Autodesk Inventor part; units mm, degrees
ref_plane "YZ Plane" through (0, 0, 0) normal (1, 0, 0) x (0, 1, 0)
ref_plane "XZ Plane" through (0, 0, 0) normal (0, 1, 0) x (-1, 0, 0)
ref_plane "XY Plane" through (0, 0, 0) normal (0, 0, 1) x (1, 0, 0)
sketch "Sketch1" plane through (0, 0, 0) normal (0, 0, 1) x (1, 0, 0)
  line L0 (-12.7, -25.4) -> (12.7, -25.4)
  line L1 (12.7, -25.4) -> (12.7, 25.4)
  line L2 (12.7, 25.4) -> (-12.7, 25.4)
  line L3 (-12.7, 25.4) -> (-12.7, -25.4)
  line L4 (-12.7, -25.4) -> (12.7, 25.4) construction
  line L5 (12.7, -25.4) -> (-12.7, 25.4) construction
  line L6 (-11.1125, 23.8125) -> (11.1125, 23.8125)
  line L7 (11.1125, 23.8125) -> (11.1125, -23.8125)
  line L8 (11.1125, -23.8125) -> (-11.1125, -23.8125)
  line L9 (-11.1125, -23.8125) -> (-11.1125, 23.8125)
  point P0 (0, 0)
  dimension "width" = 25.4
  dimension "height" = 50.8
  dimension "thickness" = 1.5875
extrude "Extrusion1" add sketch "Sketch1" along normal mid plane 914.4
sketch "Sketch2" plane through (-12.7, 25.4, 457.2) normal (0, 1, 0) x (1, 0, 0)
  line L0 (25.4, 0) -> (0, 0)
  line L1 (0, 914.4) -> (0, 0)
  point P0 (12.7, 457.2)
  point P1 (12.7, 6.35)
  point P2 (12.7, 12.7)
  point P3 (12.7, 19.05)
  point P4 (12.7, 0)
  point P5 (12.7, 0)
  dimension "d5" = 6.35
  dimension "d6" = 6.35
  dimension "d7" = 6.35
hole "Hole1" at (0, 25.4, 450.85) at (0, 25.4, 444.5) at (0, 25.4, 438.15) direction (0, -1, 0) diameter 5.1054 end through all
sketch "Sketch3" plane through (-12.7, -25.4, 457.2) normal (-1, 0, 0) x (0, 0, 1)
  line L0 (-914.4, 0) -> (-914.4, 50.8)
  point P0 (-457.2, 25.4)
  point P1 (-901.7, 38.1)
  point P2 (-901.7, 25.4)
  point P3 (-901.7, 12.7)
  point P4 (-914.4, 25.4)
  dimension "d15" = 12.7
  dimension "d16" = 12.7
  dimension "d17" = 12.7
hole "Hole2" at (-12.7, 12.7, -444.5) at (-12.7, 0, -444.5) at (-12.7, -12.7, -444.5) direction (1, 0, 0) diameter 5.1054 end through all
sketch "Sketch4" plane through (-12.7, 25.4, 457.2) normal (0, 1, 0) x (1, 0, 0)
  circle A0 centre (12.7, 19.05) radius 2.5527
  line L0 (25.4, 914.4) -> (25.4, 0)
  point P0 (12.7, 457.2)
  point P1 (15.4686, 44.45)
  dimension "d34" = 9.9314
  dimension "d55" = 25.4
hole "Hole3" at (2.7686, 25.4, 412.75) direction (0, -1, 0) diameter 9.525 end through all
sketch "Sketch5" plane through (-12.7, 25.4, 457.2) normal (0, 1, 0) x (1, 0, 0)
  line L0 (0, 914.4) -> (25.4, 914.4)
  line L1 (0, 914.4) -> (0, 0)
  point P0 (12.7, 457.2)
  point P1 (9.9314, 869.95)
  point P2 (12.7, 914.4)
  dimension "d35" = 44.45
  dimension "d36" = 9.9314
hole "Hole4" at (-2.7686, 25.4, -412.75) direction (0, -1, 0) diameter 9.525 end through all
sketch "Sketch6" plane through (12.7, -25.4, 457.2) normal (1, 0, 0) x (0, 0, -1)
  line L0 (58.42, 41.275) -> (30.48, 41.275)
  line L1 (30.48, 41.275) -> (30.48, 9.525)
  line L2 (30.48, 9.525) -> (58.42, 9.525)
  line L3 (58.42, 9.525) -> (58.42, 41.275)
  line L4 (58.42, 41.275) -> (30.48, 9.525) construction
  line L5 (30.48, 41.275) -> (58.42, 9.525) construction
  line L6 (0, 0) -> (0, 50.8)
  line L7 (914.4, 50.8) -> (0, 50.8)
  point P0 (457.2, 25.4)
  point P1 (44.45, 25.4)
  point P2 (0, 25.4)
  dimension "d44" = 30.48
  dimension "d45" = 27.94
  dimension "d47" = 31.75
extrude "Extrusion2" cut sketch "Sketch6" against normal blind 1.5875
sketch "Sketch7" plane through (-12.7, -25.4, 457.2) normal (-1, 0, 0) x (0, 0, 1)
  line L0 (-883.92, 9.525) -> (-855.98, 9.525)
  line L1 (-855.98, 9.525) -> (-855.98, 41.275)
  line L2 (-855.98, 41.275) -> (-883.92, 41.275)
  line L3 (-883.92, 41.275) -> (-883.92, 9.525)
  line L4 (-883.92, 9.525) -> (-855.98, 41.275) construction
  line L5 (-855.98, 9.525) -> (-883.92, 41.275) construction
  line L6 (-914.4, 0) -> (-914.4, 50.8)
  point P0 (-457.2, 25.4)
  point P1 (-869.95, 25.4)
  point P2 (-914.4, 25.4)
  dimension "d50" = 30.48
  dimension "d51" = 31.75
  dimension "d52" = 27.94
extrude "Extrusion3" cut sketch "Sketch7" against normal blind 1.5875
properties part number "EL2-004" material "Aluminum 6061"
Work out the finished part from the listing and answer in its coordinate system (mm). A direction names the side the tool comes from. Give positions to 0.01 mm unless a question says otherwise; leave off trailing zeros. Write each loop counter-clockwise with the first axis right and the second up, starting at its lowest first coordinate (ties: lowest second). Pieces come first, ordered by that corner, then holes.
Q1. For a pull along Y with two mould halves and no side action, classify faces 1 (the face through (0, 25.4, -6)), 2 (the face through (-11.3, 2, -457.2)), 3 (the face through (-11.112, 0, -6)) as released by +Y, released by -Y, zero draft, split by the parting line, or undercut.
Answer:
face 1: released by +Y
face 2: zero draft
face 3: undercut
Q2. A tool of negligible diameter and unlimited length cuts with its end or side. For faces 4 (the face through (-11.3, 2, 457.2)), 5 (the face through (11.112, 0, -6)), from which of +Z, -Z, +X, -X, +Y, -Y can it reach the whole face along a straight path? Write none if from no direction.
Answer:
face 4: +Z, +X, -X, +Y, -Y
face 5: +Z, -Z
Q3. Straight lines are drawn through the part: L1, parallel to Z at x = -12.1, y = 0; L2, parallel to Z at x = 11.5, y = -12.7; L3, parallel to Y at x = -11.45, z = -444.5. For each, find the intervals that lie inside material, in ascending order.
Answer:
L1: z = -457.2 to -447.05, -441.95 to -426.72, -398.78 to 457.2
L2: z = -457.2 to -447.05, -441.95 to 398.78, 426.72 to 457.2
L3: y = -25.4 to -15.25, -10.15 to -2.55, 2.55 to 10.15, 15.25 to 25.4
Q4. The part is cut by section A-A on z = 228. Give the vertices of the cut face in (x, y).
Answer:
outline: (-12.7, -25.4) - (12.7, -25.4) - (12.7, 25.4) - (-12.7, 25.4) - close; hole (-11.11, -23.81) - (11.11, -23.81) - (11.11, 23.81) - (-11.11, 23.81) - close
